```python
from build123d import *

# Parameters (mm, degrees)
SKETCH1_W           = 30
SKETCH1_H           = 30
BOSS_EXTRUDE2_DEPTH = 15
SKETCH2_R           = 15
BOSS_EXTRUDE3_DEPTH = 10
SKETCH3_R           = 15
BOSS_EXTRUDE4_DEPTH = 10
SKETCH4_R           = 9.528333781
CUT_EXTRUDE1_DEPTH  = 31
BOSS_EXTRUDE5_START = -30
SKETCH5_R           = 9.528333781
BOSS_EXTRUDE5_DEPTH = 130


with BuildPart() as part:
    # Sketch1 → Boss-Extrude2 (new body, symmetric)
    with BuildSketch(Plane.XY):
        Rectangle(SKETCH1_W, SKETCH1_H)
    extrude(amount=BOSS_EXTRUDE2_DEPTH, both=True)

    # Sketch2 → Boss-Extrude3 (add)
    with BuildSketch(Plane.XY.offset(15)):
        Circle(SKETCH2_R)
    extrude(amount=BOSS_EXTRUDE3_DEPTH)

    # Sketch3 → Boss-Extrude4 (add)
    with BuildSketch(Plane(origin=(0, 0, -15), x_dir=(-1, 0, 0), z_dir=(0, 0, -1))):
        Circle(SKETCH3_R)
    extrude(amount=BOSS_EXTRUDE4_DEPTH)

    # Sketch4 → Cut-Extrude1 (cut, through all)
    with BuildSketch(Plane(origin=(0, 15, 0), x_dir=(1, 0, 0), z_dir=(0, 1, 0))):
        Circle(SKETCH4_R)
    extrude(amount=-CUT_EXTRUDE1_DEPTH, mode=Mode.SUBTRACT)

    # Sketch5 → Boss-Extrude5 (add)
    with BuildSketch(Plane(origin=(0, 15, 0), x_dir=(1, 0, 0), z_dir=(0, 1, 0)).offset(BOSS_EXTRUDE5_START)):
        Circle(SKETCH5_R)
    extrude(amount=BOSS_EXTRUDE5_DEPTH)


solid = part.part
```
Input: part model. Units: mm. Frame: model coordinates. A direction names the side the tool comes from. Give positions to 0.01 mm unless a question says otherwise; leave off trailing zeros. Loops run counter-clockwise (first coordinate to the right, second up) from the corner with the lowest first, then second, coordinate; pieces in that order, holes last.
1) Reachability of faces 1 (the flat face through (-12, 11, -15)), 2 (the flat face through (-7, 15, 7)), 3 (the cylindrical face through (-14.985, 0.66, 19.93)) from +Z, -Z, +X, -X, +Y, -Y: full face, straight path, thin tool, end or side. Return the list, or none.
A:
face 1: -Z, -X, +Y
face 2: +Y
face 3: +Z
2) Contact query for flat-ended pins moving along their axis: pin 1 (12 mm diameter, centred on y = 99, z = -11.5, fed in from -X); pin 2 (1.5 mm diameter, centred on x = -5, z = 13.5, fed in from +Y); pin 3 (4 mm diameter, centred on y = 93.5, z = -0.5, fed in from +X). Output: stop coordinate, or through.
A:
pin 1: stops at x = -7.78
pin 2: stops at y = 15
pin 3: stops at x = 9.53
3) Section query D-D on x = -7. Return the cut outline in (y, z), and give its area (3 significant figures).
A:
outline: (-15, -15) - (-13.27, -15) - (-13.27, -25) - (13.27, -25) - (13.27, -15) - (15, -15) - (15, -6.46) - (115, -6.46) - (115, 6.46) - (15, 6.46) - (15, 15) - (13.27, 15) - (13.27, 25) - (-13.27, 25) - (-13.27, 15) - (-15, 15) - close
area: 2,720 mm2
4) Section query A-A on z = 0. Return the cut outline in (x, y).
A:
outline: (-15, -15) - (15, -15) - (15, 15) - (9.53, 15) - (9.53, 115) - (-9.53, 115) - (-9.53, 15) - (-15, 15) - close
5) Section query B-B on y = 11.5. Return the cut outline in (x, z).
A:
outline: (-15, -15) - (-9.63, -15) - (-9.63, -25) - (9.63, -25) - (9.63, -15) - (15, -15) - (15, 15) - (9.63, 15) - (9.63, 25) - (-9.63, 25) - (-9.63, 15) - (-15, 15) - close
6) Line query: L1, parallel to Y at x = 0.5, z = -14; L2, parallel to Z at x = -4.75, y = 22; L3, parallel to X at y = 30, z = 8. Output: solid intervals per line, ascending.
A:
L1: y = -15 to 15
L2: z = -8.26 to 8.26
L3: x = -5.18 to 5.18
7) Section query C-C on x = 5.25. Return the cut outline in (y, z), and give its area (3 significant figures).
A:
outline: (-15, -15) - (-14.05, -15) - (-14.05, -25) - (14.05, -25) - (14.05, -15) - (15, -15) - (15, -7.95) - (115, -7.95) - (115, 7.95) - (15, 7.95) - (15, 15) - (14.05, 15) - (14.05, 25) - (-14.05, 25) - (-14.05, 15) - (-15, 15) - close
area: 3,050 mm2
